```python
from build123d import *

# Parameters (mm, degrees)
SKETCH_1_R          = 4
SKETCH_1_R_2        = 2
EXTRUDE_1_DEPTH     = 3
SKETCH_2_R          = 3.6
SKETCH_2_R_2        = 2.5
CUT_EXTRUDE_1_DEPTH = 0.1
SKETCH_3_R          = 3.6
SKETCH_3_R_2        = 2.5
CUT_EXTRUDE_2_DEPTH = 0.1


with BuildPart() as part:
    # Эскиз1 → Бобышка-Вытянуть1 (new body)
    with BuildSketch(Plane(origin=(0, 0, 0), x_dir=(1, 0, 0), z_dir=(0, 1, 0))):
        Circle(SKETCH_1_R)
        Circle(SKETCH_1_R_2, mode=Mode.SUBTRACT)
    extrude(amount=EXTRUDE_1_DEPTH)

    # Эскиз2 → Вырез-Вытянуть1 (cut)
    with BuildSketch(Plane(origin=(0, 3, 0), x_dir=(1, 0, 0), z_dir=(0, 1, 0))):
        Circle(SKETCH_2_R)
        Circle(SKETCH_2_R_2, mode=Mode.SUBTRACT)
    extrude(amount=-CUT_EXTRUDE_1_DEPTH, mode=Mode.SUBTRACT)

    # Эскиз3 → Вырез-Вытянуть2 (cut)
    with BuildSketch(Plane.XZ):
        Circle(SKETCH_3_R)
        Circle(SKETCH_3_R_2, mode=Mode.SUBTRACT)
    extrude(amount=-CUT_EXTRUDE_2_DEPTH, mode=Mode.SUBTRACT)


solid = part.part
```
For this review, take the finished solid that the model builds, in its own axes (mm). A direction names the side the tool comes from. Round coordinates to 2 decimals unless told otherwise and drop trailing zeros. Write each loop counter-clockwise with the first axis right and the second up, starting at its lowest first coordinate (ties: lowest second). Pieces come first, ordered by that corner, then holes. Notation, with made-up numbers: (45.25, -13) -> (87.25, -13) arc R18 cw to (87.25, -3) -> close; hole circle Ø11 at (67, 46.5). An arc over 180 degrees is marked (long way). Use one line per item in the form item = value.
1) Take a section at D-D, the plane z = 3.25. Write out the cut boundary in (x, y), and give its area (3 significant figures).
Found:
outline = (-2.33, 0) -> (-1.55, 0) -> (-1.55, 0.1) -> (1.55, 0.1) -> (1.55, 0) -> (2.33, 0) -> (2.33, 3) -> (1.55, 3) -> (1.55, 2.9) -> (-1.55, 2.9) -> (-1.55, 3) -> (-2.33, 3) -> close
area = 13.4 mm2
2) Take a section at C-C, the plane y = 2.4. Write out the cut boundary in (x, z), and give its area (3 significant figures).
Found:
outline = circle Ø8 at (0, 0); hole circle Ø4 at (0, 0)
area = 37.7 mm2
3) Take a section at A-A, the plane z = 0. Write out the cut boundary in (x, y), and give its area (3 significant figures).
Found:
outline = (-4, 0) -> (-3.6, 0) -> (-3.6, 0.1) -> (-2.5, 0.1) -> (-2.5, 0) -> (-2, 0) -> (-2, 3) -> (-2.5, 3) -> (-2.5, 2.9) -> (-3.6, 2.9) -> (-3.6, 3) -> (-4, 3) -> close; (2, 0) -> (2.5, 0) -> (2.5, 0.1) -> (3.6, 0.1) -> (3.6, 0) -> (4, 0) -> (4, 3) -> (3.6, 3) -> (3.6, 2.9) -> (2.5, 2.9) -> (2.5, 3) -> (2, 3) -> close
area = 11.6 mm2
4) Tool access review of faces 5 (the flat face through (-1, 3, -2)), 6 (the flat face through (-0.9, 2.9, -2.5)): name each direction out of +Z, -Z, +X, -X, +Y, -Y from which nothing blocks a thin tool from reaching the whole face with its end or side.
Found:
face_5 = +Z, -Z, +X, -X, +Y
face_6 = +Y
5) Mouldability with a two-part tool opening along Z and no side actions: class faces 1 (the flat face through (-0.9, 0.1, 2.5)), 2 (the cylindrical face through (-0.867, 1.479, 3.905)), 3 (the flat face through (-1, 0, -2)), 4 (the cylindrical face through (0, 1, 2)) as +Z half, -Z half, draft (parallel to the pull), parting line (faces both ways), or undercut.
Found:
face_1 = undercut
face_2 = parting line
face_3 = draft
face_4 = undercut
6) Clearance check with a flat-ended pin moving along its axis: pin 1 (1 mm diameter, centred on x = 2.5, y = 2, fed in from +Z). State where the tip first meets the part, or that it passes through.
Found:
pin_1 = 3.46
7) Take a section at B-B, the plane x = 0. Write out the cut boundary in (y, z), and give its area (3 significant figures).
Found:
outline = (0, -4) -> (3, -4) -> (3, -3.6) -> (2.9, -3.6) -> (2.9, -2.5) -> (3, -2.5) -> (3, -2) -> (0, -2) -> (0, -2.5) -> (0.1, -2.5) -> (0.1, -3.6) -> (0, -3.6) -> close; (0, 2) -> (3, 2) -> (3, 2.5) -> (2.9, 2.5) -> (2.9, 3.6) -> (3, 3.6) -> (3, 4) -> (0, 4) -> (0, 3.6) -> (0.1, 3.6) -> (0.1, 2.5) -> (0, 2.5) -> close
area = 11.6 mm2
8) To check wall thickness, follow L1, parallel to Z at x = 0, y = 0.05; L2, parallel to Z at x = 0, y = 1.2. State the ranges of each line that lie inside material, in increasing order. Write a range as from..to.
Found:
L1 = -4..-3.6, -2.5..-2, 2..2.5, 3.6..4
L2 = -4..-2, 2..4
